Model file for the job. Use its own axes, mm. Round coordinates to 2 decimals unless told otherwise and drop trailing zeros. Loops run counter-clockwise (first coordinate to the right, second up) from the corner with the lowest first, then second, coordinate; pieces in that order, holes last.
Autodesk Inventor part; units mm, degrees
ref_plane "YZ Plane" through (0, 0, 0) normal (1, 0, 0) x (0, 1, 0)
ref_plane "XZ Plane" through (0, 0, 0) normal (0, 1, 0) x (-1, 0, 0)
ref_plane "XY Plane" through (0, 0, 0) normal (0, 0, 1) x (1, 0, 0)
sketch "Sketch1" plane through (0, 0, 0) normal (0, 0, 1) x (1, 0, 0)
  line L0 (-20.7908, 24.2777) -> (30.0092, 24.2777)
  line L1 (30.0092, 24.2777) -> (30.0092, -83.6723)
  line L2 (30.0092, -83.6723) -> (-20.7908, -83.6723)
  line L3 (-20.7908, -83.6723) -> (-20.7908, 24.2777)
  line L4 (26.8342, 24.2777) -> (26.8342, -1.1223)
  line L5 (26.8342, -1.1223) -> (30.0092, -1.1223)
  line L6 (26.8342, -83.6723) -> (26.8342, -58.2723)
  line L7 (26.8342, -58.2723) -> (30.0092, -58.2723)
  point P0 (0, 0)
  point P1 (-8.0908, 11.5777)
  point P2 (17.3092, 11.5777)
  point P3 (-8.0908, -70.9723)
  point P4 (17.3092, -70.9723)
  point P5 (-8.0908, -7.4723)
  point P6 (-8.0908, -15.4098)
  point P7 (-8.0908, -23.3473)
  point P8 (-8.0908, -31.2848)
  point P9 (-8.0908, -39.2223)
  point P10 (-8.0908, -47.1598)
  dimension "d0" = 50.8
  dimension "d1" = 107.95
  dimension "d2" = 12.7
  dimension "d3" = 12.7
  dimension "d4" = 12.7
  dimension "d5" = 12.7
  dimension "d6" = 12.7
  dimension "d7" = 12.7
  dimension "d8" = 12.7
  dimension "d9" = 12.7
  dimension "d12" = 7.9375
  dimension "d13" = 7.9375
  dimension "d14" = 7.9375
  dimension "d15" = 7.9375
  dimension "d16" = 7.9375
  dimension "d36" = 38.1
  dimension "d37" = 38.1
  dimension "d38" = 38.1
  dimension "d39" = 38.1
  dimension "d40" = 19.05
  dimension "d41" = 38.1
  dimension "d43" = 38.1
  dimension "d44" = 25.4
  dimension "d45" = 3.175
  dimension "d46" = 25.4
  dimension "d47" = 3.175
extrude "Extrusion1" add sketch "Sketch1" against normal blind 3.175
hole "Hole1" at (-8.0908, 11.5777, 0) at (17.3092, 11.5777, 0) at (-8.0908, -70.9723, 0) at (17.3092, -70.9723, 0) direction (0, 0, -1) diameter 6.35 depth 25.4 tip angle 118
hole "Hole2" at (-8.0908, -7.4723, 0) at (-8.0908, -15.4098, 0) at (-8.0908, -23.3473, 0) at (-8.0908, -31.2848, 0) at (-8.0908, -39.2223, 0) at (-8.0908, -47.1598, 0) direction (0, 0, -1) diameter 4.7625 depth 25.4 tip angle 118
properties part number "AS2-8-4-001"
Q1. Probe line 1 (X direction, y = 14.5, z = -2.25); line 2 (Y direction, x = -5.5, z = -2.75); line 3 (X direction, y = 10.5, z = -0.2). List the from-to ranges inside material, lowest first.
Q2. Slice it at A-A on y = -14. Give the cut face in (x, z) (3 decimals), plus the area to 3 significant figures.
Q3. Pull direction X, two halves, no side cores. Call faces 1 (the face through (30.009, -29, -2)), 2 (the face through (14.16, 11.99, -1.61)), 3 (the face through (4, 24.278, -2)): pulls with the +X half, pulls with the -X half, needs draft (parallel to the pull), parting line crosses it, or undercut.
Q4. Slice it at B-B on z = -0.85. State how many separate pieces and enclosed holes the cut face has, plus the area to 3 significant figures.
Q5. Flat gauge pin, fed straight in: P1, Ø4.5, axis at x = -8.09, y = -39.22, coming from the +Z side. Where does the tip first touch, or does it go through?
Reply:
1. line 1: x = -20.79 to -9.33, -6.85 to 16.07, 18.55 to 30.01
1. line 2: y = -83.67 to -72.81, -69.14 to 9.74, 13.41 to 24.28
1. line 3: x = -20.79 to -11.08, -5.1 to 14.32, 20.3 to 30.01
2. outline: (-20.791, -3.175) - (-10.01, -3.175) - (-10.01, 0) - (-20.791, 0) - close; (-6.172, -3.175) - (30.009, -3.175) - (30.009, 0) - (-6.172, 0) - close
2. area: 149 mm2
3. face 1: pulls with the +X half
3. face 2: undercut
3. face 3: needs draft
4. separate pieces: 1
4. enclosed holes: 10
4. area: 5,250 mm2
5. P1: passes through
